```python
from build123d import *

# Parameters (mm, degrees)
F0_W     = 40
F0_H     = 40
F1_DEPTH = 10
F2_W     = 100
F2_H     = 10
F3_DEPTH = 690
F4_W     = 100
F4_H     = 10
F5_DEPTH = 690


with BuildPart() as f1:
    # F0 (on Top) → F1 (new body, symmetric)
    with BuildSketch(Plane.XY):
        Polygon((20, -5), (50, -5), (50, 5), (20, 5), (-20, 5), (-50, 5), (-50, -5), (-20, -5), align=None)
        with Locations((0, 25)):
            Rectangle(F0_W, F0_H)
        with Locations((0, -25)):
            Rectangle(F0_W, F0_H)
        Polygon((-20, 45), (20, 45), (50, 45), (50, 55), (-50, 55), (-50, 45), align=None)
        Polygon((50, -45), (20, -45), (-20, -45), (-50, -45), (-50, -55), (50, -55), align=None)
    extrude(amount=F1_DEPTH, both=True)

    # F2 (on face) → F3 (join)
    with BuildSketch(Plane(origin=(0, 0, -10), x_dir=(1, 0, 0), z_dir=(0, 0, -1))):
        Rectangle(F2_W, F2_H)
        with Locations((0, 50)):
            Rectangle(F2_W, F2_H)
        with Locations((0, -50)):
            Rectangle(F2_W, F2_H)
    extrude(amount=F3_DEPTH)

    # F4 (on face) → F5 (join)
    with BuildSketch(Plane.XY.offset(10)):
        with Locations((0, 50)):
            Rectangle(F4_W, F4_H)
        Rectangle(F4_W, F4_H)
        with Locations((0, -50)):
            Rectangle(F4_W, F4_H)
    extrude(amount=F5_DEPTH)


solid = f1.part
```
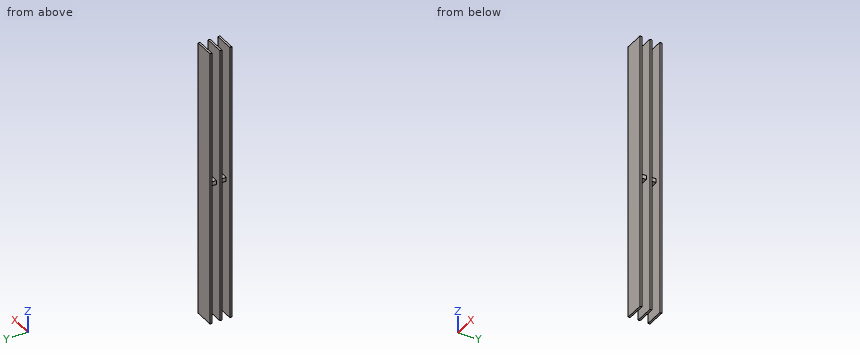
Work out the finished part from the listing and answer in its coordinate system (mm). Give positions to 0.01 mm unless a question says otherwise; leave off trailing zeros. Write each loop counter-clockwise with the first axis right and the second up, starting at its lowest first coordinate (ties: lowest second). Pieces come first, ordered by that corner, then holes. Notation, with made-up numbers: (-26, 47) -> (21, 47) arc R25 ccw to (21, 78) -> close; hole circle Ø2 at (58, -21.75). An arc over 180 degrees is marked (long way). Write item = value, one per line.
Q1. Flat-ended cylindrical pins translate along their axes: pin 1 Ø6 at (y, z) = (27.5, 4.5) entering from +X; pin 2 Ø10 at (y, z) = (-17.5, -4.5) entering from -X; pin 3 Ø20 at (x, y) = (3, -16) entering from -Z. Find the tip coordinate at first contact, or state that the pin passes through.
Computed values:
pin_1 = 20
pin_2 = -20
pin_3 = -10
Q2. Section B-B on x = -2 is taken. Determine the outline of the cut face in (y, z), and give its area (3 significant figures).
Computed values:
outline = (-55, -700) -> (-45, -700) -> (-45, -10) -> (-5, -10) -> (-5, -700) -> (5, -700) -> (5, -10) -> (45, -10) -> (45, -700) -> (55, -700) -> (55, 700) -> (45, 700) -> (45, 10) -> (5, 10) -> (5, 700) -> (-5, 700) -> (-5, 10) -> (-45, 10) -> (-45, 700) -> (-55, 700) -> close
area = 43,600 mm^2
Q3. Consider line 1 along Y through (x, z) = (43, 525.5); line 2 along Z through (x, y) = (-10, 8). Determine where each line is inside the solid, lowest interval first.
Computed values:
line_1 = -55 to -45, -5 to 5, 45 to 55
line_2 = -10 to 10
Q4. Section C-C on y = 29 is taken. Determine the outline of the cut face in (x, z).
Computed values:
outline = (-20, -10) -> (20, -10) -> (20, 10) -> (-20, 10) -> close
Q5. Section A-A on z = 502 is taken. Determine the outline of the cut face in (x, y).
Computed values:
outline = (-50, -55) -> (50, -55) -> (50, -45) -> (-50, -45) -> close; (-50, -5) -> (50, -5) -> (50, 5) -> (-50, 5) -> close; (-50, 45) -> (50, 45) -> (50, 55) -> (-50, 55) -> close
